from build123d import *
from build123d.topology import SkipClean

# Parameters (mm, degrees)
SKETCH1_W           = 50
SKETCH1_H           = 10
BOSS_EXTRUDE1_DEPTH = 70
SKETCH2_W           = 50
SKETCH2_H           = 4
CUT_EXTRUDE1_DEPTH  = 60
SKETCH3_W           = 100
SKETCH3_H           = 6
BOSS_EXTRUDE2_DEPTH = 20
FILLET1_R           = 10
FILLET2_R           = 10
FILLET3_R           = 5
CUT_EXTRUDE2_DEPTH  = 85.976467331
FILLET4_R           = 4
FILLET5_R           = 4


# Some blends are built 0.0001 mm under size
with BuildPart() as part:
    # Sketch1 → Boss-Extrude1 (new body)
    with BuildSketch(Plane(origin=(0, 0, 0), x_dir=(1, 0, 0), z_dir=(0, 1, 0))):
        Rectangle(SKETCH1_W, SKETCH1_H)
    extrude(amount=BOSS_EXTRUDE1_DEPTH)

    # Sketch2 → Cut-Extrude1 (cut)
    with BuildSketch(Plane(origin=(0, 70, 0), x_dir=(1, 0, 0), z_dir=(0, 1, 0))):
        Rectangle(SKETCH2_W, SKETCH2_H)
    extrude(amount=-CUT_EXTRUDE1_DEPTH, mode=Mode.SUBTRACT)

    # Sketch3 → Boss-Extrude2 (add)
    with BuildSketch(Plane.XY.offset(5)):
        with Locations((0, 3)):
            Rectangle(SKETCH3_W, SKETCH3_H)
    extrude(amount=BOSS_EXTRUDE2_DEPTH)

    # Fillet1
    fillet1_edges = [part.edges().sort_by_distance(p)[0] for p in [
        (50, 3, 25),
        (-50, 3, 25),
        (-50, 3, 5),
        (50, 3, 5),
    ]]
    fillet(fillet1_edges, radius=FILLET1_R - 0.0001)  # a hair under: the kernel refuses the full size

    # Fillet2
    fillet2_edges = [part.edges().sort_by_distance(p)[0] for p in [
        (-25, 3, 5),
        (25, 3, 5),
    ]]
    fillet(fillet2_edges, radius=FILLET2_R - 0.0001)  # a hair under: the kernel refuses the full size

    # Fillet3
    # the kernel refuses this fillet: 5 mm, written as the material it adds along each edge
    with BuildSketch(Plane(origin=(-25, 6, 5), x_dir=(-1, 0, 0), z_dir=(0, 0, -1))) as fillet3_piece_1_section:
        with BuildLine():
            CenterArc((FILLET3_R, FILLET3_R), FILLET3_R, 180, 90)
            Line((0, FILLET3_R), (0, 0))
            Line((0, 0), (FILLET3_R, 0))
        make_face()
    fillet3_piece_1 = extrude(amount=22.4999, mode=Mode.PRIVATE)
    fillet3_piece_1 = fillet3_piece_1 - Plane(origin=(-34.9999, 7.107412722, -4.9999), x_dir=(0, 0, 1), z_dir=(0, 1, 0)) * Cylinder(9.9999, 65, mode=Mode.PRIVATE)
    fillet3_piece_1 = split(fillet3_piece_1, bisect_by=Plane(origin=(-26.097313128, 7.107412722, -5), z_dir=(0, 0, 1)), keep=Keep.TOP, mode=Mode.PRIVATE)
    fillet3_piece_1 = split(fillet3_piece_1, bisect_by=Plane(origin=(-26.097313128, 10, 3.51164162), z_dir=(0, -1, 0)), keep=Keep.TOP, mode=Mode.PRIVATE)
    add(fillet3_piece_1)
    with BuildSketch(Plane(origin=(-25, 6, 5), x_dir=(-1, 0, 0), z_dir=(0, 0, -1))) as fillet3_piece_2_section:
        with BuildLine():
            CenterArc((FILLET3_R, FILLET3_R), FILLET3_R, 180, 90)
            Line((0, FILLET3_R), (0, 0))
            Line((0, 0), (FILLET3_R, 0))
        make_face()
    fillet3_piece_2 = extrude(amount=22.4999, mode=Mode.PRIVATE)
    fillet3_piece_2 = split(fillet3_piece_2, bisect_by=Plane(origin=(-25.030252938, 10, 3.5), z_dir=(0, 1, 0)), keep=Keep.TOP, mode=Mode.PRIVATE)
    fillet3_piece_2 = split(fillet3_piece_2, bisect_by=Plane(origin=(-25.030252938, 10.249492121, 2), z_dir=(0, 0, 1)), keep=Keep.TOP, mode=Mode.PRIVATE)
    add(fillet3_piece_2)
    with BuildSketch(Plane(origin=(-25, 6, 17.5), x_dir=(-1, 0, 0), z_dir=(0, 0, -1))) as fillet3_piece_3_section:
        with BuildLine():
            CenterArc((FILLET3_R, FILLET3_R), FILLET3_R, 180, 90)
            Line((0, FILLET3_R), (0, 0))
            Line((0, 0), (FILLET3_R, 0))
        make_face()
    fillet3_piece_3 = extrude(amount=34.9999, mode=Mode.PRIVATE)
    fillet3_piece_3 = fillet3_piece_3 - Plane(origin=(-34.9999, 10.264980521, -4.9999), x_dir=(0, 0, 1), z_dir=(0, 1, 0)) * Cylinder(9.9999, 90, mode=Mode.PRIVATE)
    fillet3_piece_3 = split(fillet3_piece_3, bisect_by=Plane(origin=(-25.027128676, 10.264980521, -5), z_dir=(0, 0, 1)), keep=Keep.TOP, mode=Mode.PRIVATE)
    fillet3_piece_3 = split(fillet3_piece_3, bisect_by=Plane(origin=(-25.027128676, 10.264980521, -2), z_dir=(0, 0, -1)), keep=Keep.TOP, mode=Mode.PRIVATE)
    add(fillet3_piece_3)
    with BuildSketch(Plane(origin=(25, 6, 5), x_dir=(1, 0, 0), z_dir=(0, 0, -1))) as fillet3_piece_4_section:
        with BuildLine():
            CenterArc((FILLET3_R, -FILLET3_R), FILLET3_R, 90, 90)
            Line((0, -FILLET3_R), (0, 0))
            Line((0, 0), (FILLET3_R, 0))
        make_face()
    fillet3_piece_4 = extrude(amount=22.4999, mode=Mode.PRIVATE)
    fillet3_piece_4 = fillet3_piece_4 - Plane(origin=(34.9999, 7.107412722, -4.9999), x_dir=(0, 0, 1), z_dir=(0, 1, 0)) * Cylinder(9.9999, 65, mode=Mode.PRIVATE)
    fillet3_piece_4 = split(fillet3_piece_4, bisect_by=Plane(origin=(26.097313128, 7.107412722, -5), z_dir=(0, 0, 1)), keep=Keep.TOP, mode=Mode.PRIVATE)
    fillet3_piece_4 = split(fillet3_piece_4, bisect_by=Plane(origin=(26.097313128, 10, 3.51164162), z_dir=(0, -1, 0)), keep=Keep.TOP, mode=Mode.PRIVATE)
    add(fillet3_piece_4)
    with BuildSketch(Plane(origin=(25, 6, 5), x_dir=(1, 0, 0), z_dir=(0, 0, -1))) as fillet3_piece_5_section:
        with BuildLine():
            CenterArc((FILLET3_R, -FILLET3_R), FILLET3_R, 90, 90)
            Line((0, -FILLET3_R), (0, 0))
            Line((0, 0), (FILLET3_R, 0))
        make_face()
    fillet3_piece_5 = extrude(amount=22.4999, mode=Mode.PRIVATE)
    fillet3_piece_5 = split(fillet3_piece_5, bisect_by=Plane(origin=(25.030252938, 10, 3.5), z_dir=(0, 1, 0)), keep=Keep.TOP, mode=Mode.PRIVATE)
    fillet3_piece_5 = split(fillet3_piece_5, bisect_by=Plane(origin=(25.030252938, 10.249492121, 2), z_dir=(0, 0, 1)), keep=Keep.TOP, mode=Mode.PRIVATE)
    add(fillet3_piece_5)
    with BuildSketch(Plane(origin=(25, 6, 17.5), x_dir=(1, 0, 0), z_dir=(0, 0, -1))) as fillet3_piece_6_section:
        with BuildLine():
            CenterArc((FILLET3_R, -FILLET3_R), FILLET3_R, 90, 90)
            Line((0, -FILLET3_R), (0, 0))
            Line((0, 0), (FILLET3_R, 0))
        make_face()
    fillet3_piece_6 = extrude(amount=34.9999, mode=Mode.PRIVATE)
    fillet3_piece_6 = fillet3_piece_6 - Plane(origin=(34.9999, 10.264980521, -4.9999), x_dir=(0, 0, 1), z_dir=(0, 1, 0)) * Cylinder(9.9999, 90, mode=Mode.PRIVATE)
    fillet3_piece_6 = split(fillet3_piece_6, bisect_by=Plane(origin=(25.027128676, 10.264980521, -5), z_dir=(0, 0, 1)), keep=Keep.TOP, mode=Mode.PRIVATE)
    fillet3_piece_6 = split(fillet3_piece_6, bisect_by=Plane(origin=(25.027128676, 10.264980521, -2), z_dir=(0, 0, -1)), keep=Keep.TOP, mode=Mode.PRIVATE)
    add(fillet3_piece_6)

    # Sketch4 → Cut-Extrude2 (cut, through all)
    with SkipClean():  # the faces are left unmerged after this step: merging them gives an invalid solid
        with BuildSketch(Plane(origin=(0, 6, 0), x_dir=(1, 0, 0), z_dir=(0, 1, 0))):
            with BuildLine():
                Line((-40, -13.4), (40, -13.4))
                ThreePointArc((40, -13.4), (41.6, -15), (40, -16.6))
                Line((40, -16.6), (-40, -16.6))
                ThreePointArc((-40, -16.6), (-41.6, -15), (-40, -13.4))
            make_face()
        extrude(amount=-CUT_EXTRUDE2_DEPTH, mode=Mode.SUBTRACT)
    add(part.part.scale(1), mode=Mode.REPLACE)  # the faces are merged on a copy

    # Fillet4
    # the kernel refuses this fillet: 4 mm, written as the material it takes off along each edge
    with BuildSketch(Plane(origin=(-34.682458366, 70, 5), x_dir=(0, -1, 0), z_dir=(1, 0, 0))) as fillet4_piece_1:
        with BuildLine():
            CenterArc((3.872983346, 4), FILLET4_R, 194.477512186, 75.522487814)
            Line((0, 3), (-0.077459667, 2.98))
            ThreePointArc((-0.077459667, 2.98), (-0.08, 1.5), (-0.08, 0))
            Line((-0.08, 0), (0, -0.08))
            Line((0, -0.08), (3.872983346, -0.08))
            Line((3.872983346, -0.08), (3.872983346, 0))
        make_face()
    extrude(amount=69.364916731, mode=Mode.SUBTRACT)
    with BuildSketch(Plane(origin=(34.682458366, 70, -5), x_dir=(0, 0, 1), z_dir=(-1, 0, 0))) as fillet4_piece_2:
        with BuildLine():
            CenterArc((4, -3.872983346), FILLET4_R, 104.477512186, 75.522487814)
            Line((0, -3.872983346), (-0.08, -3.872983346))
            Line((-0.08, -3.872983346), (-0.08, 0))
            Line((-0.08, 0), (0, 0.08))
            ThreePointArc((0, 0.08), (1.5, 0.08), (2.98, 0.077459667))
            Line((2.98, 0.077459667), (3, 0))
        make_face()
    extrude(amount=69.364916731, mode=Mode.SUBTRACT)

    # Fillet5
    fillet5_edges = [part.edges().sort_by_distance(p)[0] for p in [
        (0, 6, 5),
    ]]
    fillet(fillet5_edges, radius=FILLET5_R)


solid = part.part
Design review of the part built by this model. Coordinates are the model's own, in mm. A direction names the side the tool comes from. Coordinates: 2 decimals unless noted, no trailing zeros. Order: outer loops, then holes, each group sorted by start corner. A loop starts at its lowest first (then second) coordinate and runs counter-clockwise, first axis right, second up.
Item 1: Take a section at A-A, the plane y = 56.5. Write out the cut boundary in (x, z).
Item 2: For faces 4 (the flat face through (-1, 3, 13.4)), 5 (the flat face through (0, 10, 0)), 6 (the flat face through (0, 38, 5)), 7 (the flat face through (37, 3, 5)), 8 (the flat face through (25, 42, -3)), list the 3-axis set-ups (+Z, -Z, +X, -X, +Y, -Y) from which the entire face can be reached by the end or side of a thin tool; tool diameter is ignored.
Item 3: For line 1 (Z direction, x = -17.5, y = 29); line 2 (Y direction, x = -22, z = 20.25); line 3 (X direction, y = 33, z = 2.5), list the stretches that pass through material, from the lowest coordinate up.
Item 4: Take a section at C-C, the plane x = -31.5. Write out the cut boundary in (y, z).
Item 5: Take a section at D-D, the plane z = 21. Write out the cut boundary in (x, y).
Item 6: For pin 1 Ø10 at (x, y) = (0.5, 46.5) entering from +Z; pin 2 Ø4.5 at (x, z) = (-6.5, 1) entering from +Y; pin 3 Ø1.5 at (x, y) = (-37, 3.5) entering from -Z; pin 4 Ø2.5 at (y, z) = (19.5, -3) entering from -X, all flat-tipped, find the tip position at first contact; note any pin that passes through.
Item 7: Take a section at B-B, the plane x = -3.5. Write out the cut boundary in (y, z), then the cut area to 3 significant figures.
Item 8: The part is to be moulded in two halves that separate along Z. For faces 1 (the flat face through (-38, 3, 5)), 2 (the cylindrical face through (46.99, 3.04, 22.15)), 3 (the flat face through (0, 40, 2)), say which applies: pulls with the +Z half, pulls with the -Z half, needs draft (parallel to the pull), parting line crosses it, or undercut.
The answers:
1. outline: (-25, -5) - (25, -5) - (25, -2) - (-25, -2) - close; (-25, 2) - (25, 2) - (25, 5) - (-25, 5) - close
2. face 4: +Y, -Y
2. face 5: +X, -X, +Y
2. face 6: +Z, +X, -X, +Y
2. face 7: -Z, +X, +Y, -Y
2. face 8: +Z, -Z, +X, +Y
3. line 1: z = -5 to -2, 2 to 5
3. line 2: y = 0 to 6
3. line 3: x = -25 to 25
4. outline: (0, 4.37) - (6, 4.37) - (6, 13.4) - (0, 13.4) - close; (0, 16.6) - (6, 16.6) - (6, 25) - (0, 25) - close
5. outline: (-48, 0) - (48, 0) - (48, 6) - (-48, 6) - close
6. pin 1: stops at z = 5
6. pin 2: stops at y = 70
6. pin 3: stops at z = 5
6. pin 4: stops at x = -25
7. outline: (0, -5) - (66.13, -5) arc R4 ccw to (70, -2) - (10, -2) - (10, 2) - (70, 2) arc R4 ccw to (66.13, 5) - (10, 5) arc R4 cw to (6, 9) - (6, 13.4) - (0, 13.4) - close; (0, 16.6) - (6, 16.6) - (6, 25) - (0, 25) - close
7. area: 558 mm2
8. face 1: pulls with the -Z half
8. face 2: pulls with the +Z half
8. face 3: undercut
